from build123d import *

# Parameters (mm, degrees)
F0_W     = 77.585459
F0_H     = 91.901824
F1_DEPTH = 12.46909
F2_W     = 67.887273
F2_H     = 91.439999
F3_DEPTH = 10.39091
F4_R     = 2.818603
F5_DEPTH = 18.67939
F7_DEPTH = 18.80963


with BuildPart() as f1:
    # F0 (on Front) → F1 (new body)
    with BuildSketch(Plane.XZ):
        with Locations((1.154546, -3.81)):
            Rectangle(F0_W, F0_H)
    extrude(amount=F1_DEPTH)

    # F2 (on Front) → F3 (cut)
    with BuildSketch(Plane.XZ):
        with Locations((1.154547, 0.346363)):
            Rectangle(F2_W, F2_H)
    extrude(amount=F3_DEPTH, mode=Mode.SUBTRACT)

    # F4 (on face) → F5 (join)
    with BuildSketch(Plane(origin=(0, -10.39091, 0), x_dir=(-1, 0, 0), z_dir=(0, 1, 0))):
        with Locations((21.451365, 32.264516)):
            Circle(F4_R)
        with Locations((21.451365, -35.390843)):
            Circle(F4_R)
    extrude(amount=F5_DEPTH)

    # F6 (on face) → F7 (join)
    with BuildSketch(Plane(origin=(0, -10.39091, 0), x_dir=(-1, 0, 0), z_dir=(0, 1, 0))):
        with BuildLine():
            ThreePointArc((16.163638, 24.36091), (14.893637, 25.630911), (13.623635, 24.36091))
            Line((13.623635, 24.36091), (13.623635, -28.748181))
            ThreePointArc((13.623635, -28.748181), (14.893637, -30.018182), (16.163638, -28.748181))
            Line((16.163638, -28.748181), (16.163638, 24.36091))
        make_face()
    extrude(amount=F7_DEPTH)


solid = f1.part
The listing builds one solid part. Answer for the finished solid, in the listing's coordinates (mm). A direction names the side the tool comes from. Give positions to 0.01 mm unless a question says otherwise; leave off trailing zeros. Write each loop counter-clockwise with the first axis right and the second up, starting at its lowest first coordinate (ties: lowest second). Pieces come first, ordered by that corner, then holes.
Item 1: Section D-D, the plane y = 6.25 is taken. Write down the section's boundary in (x, z), plus the area to 3 significant figures.
Item 2: Find the intervals of material crossed by line 1 along X through (y, z) = (-1.5, -10); line 2 along X through (y, z) = (-10.25, 38.5); line 3 along X through (y, z) = (5.5, 6), in increasing order.
Item 3: Flat-ended cylindrical pins translate along their axes: P1, Ø5, axis at x = -3, y = -4, coming from the +Z side; P2, Ø2, axis at y = 5.5, z = 4.5, coming from the +X side; P3, Ø5, axis at x = 2.5, z = -6, coming from the +Y side. Find the tip coordinate at first contact, or state that the pin passes through.
Item 4: Which of the six approach directions +Z, -Z, +X, -X, +Y, -Y give full straight-line access (tool end or side, diameter ignored) to faces 1 (the flat face through (-37.638, -6, -4)), 2 (the flat face through (-13.624, -1, -2)), 3 (the cylindrical face through (-14.866, -1.118, -30.018))?
Item 5: Section A-A, the plane z = -16 is taken. Write down the section's boundary in (x, y), plus the area to 3 significant figures.
Item 6: Section B-B, the plane x = 30 is taken. Write down the section's boundary in (y, z), plus the area to 3 significant figures.
Item 7: Section C-C, the plane y = -7.5 is taken. Write down the section's boundary in (x, z), plus the area to 3 significant figures.
Item 8: Determine the mould class of faces 4 (the flat face through (39.947, -6, -4)), 5 (the flat face through (1, -12.469, -3)), 6 (the flat face through (1, -5, -45.374)) for opening direction X: released by +X, released by -X, zero draft, split by the parting line, or undercut.
Completed:
1. outline: circle Ø5.64 at (-21.45, -35.39); circle Ø5.64 at (-21.45, 32.26); (-16.16, -28.75) arc R1.27 ccw to (-13.62, -28.75) - (-13.62, 24.36) arc R1.27 ccw to (-16.16, 24.36) - close
1. area: 190 mm2
2. line 1: x = -37.64 to -32.79, -16.16 to -13.62, 35.1 to 39.95
2. line 2: x = -37.64 to -32.79, 35.1 to 39.95
2. line 3: x = -16.16 to -13.62
3. P1: stops at z = -45.37
3. P2: stops at x = -13.62
3. P3: stops at y = -10.39
4. face 1: +Z, -Z, -X, +Y, -Y
4. face 2: +Z, +Y
4. face 3: +Y
5. outline: (-37.64, -12.47) - (39.95, -12.47) - (39.95, 0) - (35.1, 0) - (35.1, -10.39) - (-13.62, -10.39) - (-13.62, 8.42) - (-16.16, 8.42) - (-16.16, -10.39) - (-32.79, -10.39) - (-32.79, 0) - (-37.64, 0) - close
5. area: 310 mm2
6. outline: (-12.47, -49.76) - (0, -49.76) - (0, -45.37) - (-10.39, -45.37) - (-10.39, 42.14) - (-12.47, 42.14) - close
6. area: 237 mm2
7. outline: (-37.64, -49.76) - (39.95, -49.76) - (39.95, 42.14) - (35.1, 42.14) - (35.1, -45.37) - (-32.79, -45.37) - (-32.79, 42.14) - (-37.64, 42.14) - close; circle Ø5.64 at (-21.45, -35.39); circle Ø5.64 at (-21.45, 32.26); (-16.16, -28.75) arc R1.27 ccw to (-13.62, -28.75) - (-13.62, 24.36) arc R1.27 ccw to (-16.16, 24.36) - close
7. area: 1,380 mm2
8. face 4: released by +X
8. face 5: zero draft
8. face 6: undercut
